from build123d import *

# Parameters (mm, degrees)
CROQUIS3_R              = 3.75
CROQUIS3_R_2            = 2.5
SALIENTE_EXTRUIR1_DEPTH = 22.5


with BuildPart() as part:
    # Croquis3 → Saliente-Extruir1 (new body)
    with BuildSketch(Plane.XY):
        with Locations((-1, 153.5)):
            Circle(CROQUIS3_R)
        with Locations((-1, 153.5)):
            Circle(CROQUIS3_R_2, mode=Mode.SUBTRACT)
        with BuildLine():
            Line((0, 0), (0, 149.885791926))
            ThreePointArc((0, 149.885791926), (-1, 149.75), (-2, 149.885791926))
            Line((-2, 149.885791926), (-2, 7.5))
            Line((-2, 7.5), (0, 0))
        make_face()
    extrude(amount=SALIENTE_EXTRUIR1_DEPTH)


solid = part.part
CAD build for the part. Positions are in the model's coordinates, mm. A direction names the side the tool comes from. Round coordinates to 2 decimals unless told otherwise and drop trailing zeros. Loops run counter-clockwise (first coordinate to the right, second up) from the corner with the lowest first, then second, coordinate; pieces in that order, holes last. Notation, with made-up numbers: (88.25, -35) - (104.25, -35) arc R25 ccw to (104.25, -9) - close; hole circle Ø2 at (89, 15). An arc over 180 degrees is marked (long way). Put each result on its own line as item: value.
1. Slice it at B-B on z = 6.25. List the corners of the cut face in (x, y).
Geometry check:
outline: (-2, 7.5) - (0, 0) - (0, 149.89) arc R3.75 ccw (long way) to (-2, 149.89) - close; hole circle Ø5 at (-1, 153.5)
2. Slice it at C-C on y = 53. List the corners of the cut face in (x, z).
Geometry check:
outline: (-2, 0) - (0, 0) - (0, 22.5) - (-2, 22.5) - close
3. 3-axis set-ups, long thin cutter, end or side, ignore diameter. For faces 1 (the flat face through (-1, 85, 22.5)), 2 (the flat face through (-2, 80, 11)), 3 (the flat face through (0, 74, 11)): which of +Z, -Z, +X, -X, +Y, -Y reach the whole face in a straight line?
Geometry check:
face 1: +Z, +X, -X, +Y, -Y
face 2: +Z, -Z, -X, -Y
face 3: +Z, -Z, +X, -Y
4. Slice it at A-A on y = 153.5. List the corners of the cut face in (x, z), and give its area (4 significant figures).
Geometry check:
outline: (-4.75, 0) - (-3.5, 0) - (-3.5, 22.5) - (-4.75, 22.5) - close; (1.5, 0) - (2.75, 0) - (2.75, 22.5) - (1.5, 22.5) - close
area: 56.25 mm²
5. Pin check, flat tips, straight feed: P1, Ø11, axis at y = 63.5, z = 13, coming from the -X side; P2, Ø1.5, axis at x = 2, z = 4, coming from the -Y side; P3, Ø2, axis at x = 2, z = 6.5, coming from the +Y side. Stop position of each tip, or through.
Geometry check:
P1: x = -2
P2: y = 150.5
P3: y = 156.67
6. Two-plate mould, pull along Y, no slides. Class faces 4 (the cylindrical face through (-1, 156, 11)), 5 (the flat face through (-1.014, 3.802, 11.092)), 6 (the cylindrical face through (-0.849, 157.247, 11.092)), 7 (the flat face through (-1, 85, 0)): released by +Y, released by -Y, zero draft, split by the parting line, or undercut.
Geometry check:
face 4: undercut
face 5: released by -Y
face 6: split by the parting line
face 7: zero draft
7. Wall check: line 1 (X direction, y = 153.5, z = 8); line 2 (X direction, y = 131, z = 13.5); line 3 (Y direction, x = -3, z = 5). Give the ranges that are in metal, low to high.
Geometry check:
line 1: -4.75 to -3.5, 1.5 to 2.75
line 2: -2 to 0
line 3: 150.33 to 152, 155 to 156.67
